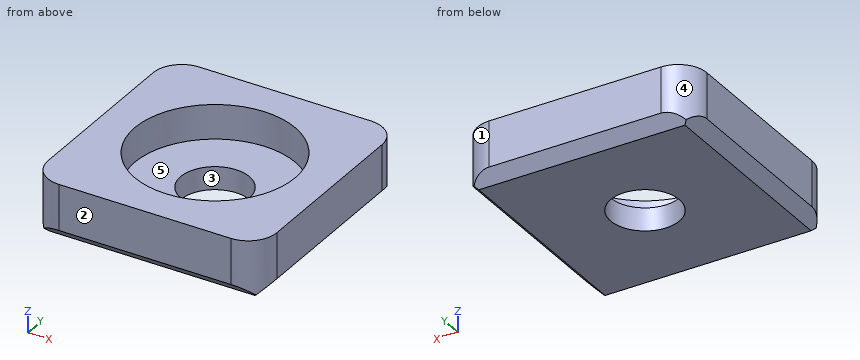
Autodesk Inventor part; units mm, degrees
ref_plane "YZ Plane" through (0, 0, 0) normal (1, 0, 0) x (0, 1, 0)
ref_plane "XZ Plane" through (0, 0, 0) normal (0, 1, 0) x (-1, 0, 0)
ref_plane "XY Plane" through (0, 0, 0) normal (0, 0, 1) x (1, 0, 0)
sketch "Sketch1" plane through (0, 0, 0) normal (0, 0, 1) x (1, 0, 0)
  line L0 (0, 0) -> (25.4, 0)
  line L1 (25.4, 0) -> (25.4, 25.4)
  line L2 (25.4, 25.4) -> (0, 25.4)
  line L3 (0, 25.4) -> (0, 0)
  dimension "d0" = 25.4
extrude "Extrusion1" add sketch "Sketch1" along normal blind 6.35
sketch "Sketch2" plane through (0, 0, 6.35) normal (0, 0, 1) x (1, 0, 0)
  line L0 (25.4, 25.4) -> (0, 25.4) construction
  line L1 (25.4, 0) -> (25.4, 25.4) construction
  line L2 (0, 25.4) -> (25.4, 0) construction
  line L3 (0, 0) -> (25.4, 25.4) construction
  point P0 (12.7, 12.7)
hole "Hole1" at (12.7, 12.7, 6.35) direction (0, 0, -1) diameter 7.62 end through all counterbore diameter 17.78 counterbore depth 3.81
chamfer "Chamfer1" distance 1.27 angle 45 4 edges at (25.4, 12.7, 0) (12.7, 25.4, 0) (0, 12.7, 0) (12.7, 0, 0)
fillet "Fillet1" radius 3.175 4 edges at (25.4, 25.4, 3.81) (0, 25.4, 3.81) (25.4, 0, 3.81) (0, 0, 3.81)
properties part number "testpot"
Source: CAD feature listing. Evaluate the final solid. Frame: model axes, mm. Face numbers are marked on the shaded views. A direction names the side the tool comes from. Give positions to 0.01 mm unless a question says otherwise; leave off trailing zeros. Write each loop counter-clockwise with the first axis right and the second up, starting at its lowest first coordinate (ties: lowest second). Pieces come first, ordered by that corner, then holes. Notation, with made-up numbers: (28.5, -5) -> (76.5, -5) arc R25 ccw to (76.5, 10) -> close; hole circle Ø10 at (-10, 44). An arc over 180 degrees is marked (long way). Return JSON: item names as keys, results as strings. Group by question number.
1. Pin query (flat end, axial travel): pin 1 Ø9 at (x, y) = (12.7, 12.7) entering from +Z. Return the tip coordinate at first contact, or that it passes through.
2. Access query for the marked faces 4 and 5. Directions: +Z, -Z, +X, -X, +Y, -Y. A direction counts if a zero-diameter tool reaches every point of the face in a straight line with its end or side. Return the directions, or none.
3. Section D-D, the plane y = 21.25. Output: boundary loops of the cut face in (x, z), then the cut area to 3 significant figures.
4. Section B-B, the plane z = 2. Output: boundary loops of the cut face in (x, y) (3 decimals), then the cut area to 3 significant figures.
5. Material intervals for line 1 (X direction, y = 12.7, z = 5.4); line 2 (Y direction, x = 12.7, z = 1.5), sorted ascending. Write a range as from..to.
6. Section A-A, the plane y = 12.7. Output: boundary loops of the cut face in (x, z).
7. Mould query, pull axis Y, two halves, no side actions, for the marked faces 1, 2 and 3. Classes: +Y half, -Y half, draft (parallel to the pull), parting line (faces both ways), or undercut.
Determined:
{
 "1": {"pin 1": "stops at z = 2.54"},
 "2": {"face 4": "+Z, -Z, -X, +Y", "face 5": "+Z"},
 "3": {"outline": "(0, 1.27) -> (1.27, 0) -> (24.13, 0) -> (25.4, 1.27) -> (25.4, 6.35) -> (15.14, 6.35) -> (15.14, 2.54) -> (10.26, 2.54) -> (10.26, 6.35) -> (0, 6.35) -> close", "area": "141 mm2"},
 "4": {"outline": "(0, 3.175) arc R3.175 ccw to (3.175, 0) -> (22.225, 0) arc R3.175 ccw to (25.4, 3.175) -> (25.4, 22.225) arc R3.175 ccw to (22.225, 25.4) -> (3.175, 25.4) arc R3.175 ccw to (0, 22.225) -> close; hole circle Ø7.62 at (12.7, 12.7)", "area": "591 mm2"},
 "5": {"line 1": "x = 0..3.81, 21.59..25.4", "line 2": "y = 0..8.89, 16.51..25.4"},
 "6": {"outline": "(0, 1.27) -> (1.27, 0) -> (8.89, 0) -> (8.89, 2.54) -> (3.81, 2.54) -> (3.81, 6.35) -> (0, 6.35) -> close; (16.51, 0) -> (24.13, 0) -> (25.4, 1.27) -> (25.4, 6.35) -> (21.59, 6.35) -> (21.59, 2.54) -> (16.51, 2.54) -> close"},
 "7": {"face 1": "+Y half", "face 2": "-Y half", "face 3": "undercut"}
}
